Autodesk Inventor part; units mm, degrees
ref_plane "Work Plane1" through (0, -12.75, 0) normal (0, 1, 0) x (-1, 0, 0)
ref_plane "Work Plane2" through (0, -12.75, 0) normal (0, 1, 0) x (-1, 0, 0)
ref_plane "YZ Plane" through (0, 0, 0) normal (1, 0, 0) x (0, 1, 0)
sketch "Sketch1" plane through (0, 0, 0) normal (0, 0, 1) x (1, 0, 0)
  circle A0 centre (0, 0) radius 12.75
  circle A1 centre (0, 0) radius 12.25
  dimension "d0" = 25.5
  dimension "d1" = 24.5
extrude "Extrusion1" add sketch "Sketch1" along normal blind 49.5
sketch "Sketch2" plane through (0, 0, 49.5) normal (0, 0, 1) x (1, 0, 0)
  line L0 (-17.85, 0) -> (17.85, 0)
  line L1 (0, -17.85) -> (0, 17.85)
  line L2 (0, 0) -> (-12.3156, 3.2999)
  line L3 (0, 0) -> (-9.0156, -9.0156)
  line L4 (0, 0) -> (12.3156, 3.2999)
  line L5 (0, 0) -> (9.0156, -9.0156)
  arc A0 (11.8326, 3.1705) -> (-11.8326, 3.1705) centre (0, 0) ccw
  arc A1 (-8.6621, -8.6621) -> (8.6621, -8.6621) centre (0, 0) ccw
  circle A2 centre (0, 0) radius 12.75
  dimension "d4" = 15
  dimension "d5" = 45
extrude "Extrusion2" cut sketch "Sketch2" against normal blind 10 contours L5 A1 L1 | L1 A1 L3 | A1 L5 A2 L1 | L1 A2 L3 A1 | A0 L2 A2 L1 | L1 A2 L4 A0
sketch "Sketch3" plane through (0, 0, 0) normal (0, 0, -1) x (-1, 0, 0)
  circle A0 centre (0, 0) radius 12.75
extrude "Extrusion3" add sketch "Sketch3" along normal blind 1
ref_plane "Work Plane1" through (0, -12.75, 0) normal (0, 1, 0) x (-1, 0, 0)
ref_plane "Work Plane2" through (0, -12.75, 0) normal (0, 1, 0) x (-1, 0, 0)
sketch "Sketch7" plane through (0, 0, 49.5) normal (0, 0, 1) x (1, 0, 0)
  arc A0 (9.0156, -9.0156) -> (12.3156, 3.2999) centre (0, 0) ccw
  arc A1 (8.6621, -8.6621) -> (11.8326, 3.1705) centre (0, 0) ccw
  line L0 (8.6621, -8.6621) -> (9.0156, -9.0156)
  line L1 (-10.4211, -8.1317) -> (11.1081, -8.1317)
  line L2 (11.1081, -8.1317) -> (11.1081, -13.0652)
  line L3 (11.1081, -13.0652) -> (-10.4211, -13.0652)
  line L4 (-10.4211, -13.0652) -> (-10.4211, -8.1317)
extrude "Extrusion6" cut sketch "Sketch7" against normal through all
sketch "Sketch9" plane through (0, 0, 0) normal (0, 0, 1) x (1, 0, 0)
  arc A0 (9.1617, -8.1317) -> (-9.1617, -8.1317) centre (0, 0) ccw
  line L0 (-17.85, 0) -> (17.85, 0)
  point P0 (4, 0)
  dimension "d29" = 4
hole "Hole2" at (4, 0, 0) direction (0, 0, -1) diameter 1.778 depth 8 tip angle 118 countersink diameter 3.023 countersink angle 82
pattern_circular "Circular Pattern1" count 3 over 360 about axis through (0, 0, -10) along (0, 0, 1) of "Hole2"
sketch "Sketch10" plane through (0, 0, 0) normal (0, 0, 1) x (1, 0, 0)
  arc A0 (9.1617, -8.1317) -> (-9.1617, -8.1317) centre (0, 0) ccw
hole "Hole3" at (0, 0, 0) direction (0, 0, -1) diameter 1.778 end through all
properties part number "ss_inner_guide_top"
Input: part model. Units: mm. Frame: model coordinates. A direction names the side the tool comes from. Coordinates: 2 decimals unless noted, no trailing zeros. Loops run counter-clockwise (first coordinate to the right, second up) from the corner with the lowest first, then second, coordinate; pieces in that order, holes last. Notation, with made-up numbers: M 10.25,69 L 43.25,69 A15 ccw 43.25,78 Z; hole C 40,-1.75 d8. An arc over 180 degrees is marked long. Answer in a Markdown table with one row per item.
1. Section B-B, the plane x = 0. Output: boundary loops of the cut face in (y, z).
Response:
| item | result |
|---|---|
| outline | M -8.13,-1 L -0.89,-1 L -0.89,0 L -8.13,0 Z; M 0.89,-1 L 12.75,-1 L 12.75,39.5 L 12.25,39.5 L 12.25,0 L 0.89,0 Z |
2. Draft query along Y for faces 3 (the flat face through (12.1, -2.8, 49.5)), 4 (the cylindrical face through (0.404, 12.744, 24.604)), 5 (the cylindrical face through (0.87, 0.19, -0.51)), 6 (the flat face through (-9.5, -8.132, 24.4)). Return one class per face: pulls with the +Y half, pulls with the -Y half, needs draft (parallel to the pull), parting line crosses it, or undercut.
Response:
| item | result |
|---|---|
| face 3 | needs draft |
| face 4 | parting line crosses it |
| face 5 | undercut |
| face 6 | pulls with the -Y half |
3. Section C-C, the plane y = -6. Output: boundary loops of the cut face in (x, z).
Response:
| item | result |
|---|---|
| outline | M -11.25,-1 L 11.25,-1 L 11.25,49.5 L 10.68,49.5 L 10.68,0 L -10.68,0 L -10.68,49.5 L -11.25,49.5 Z |
4. Section D-D, the plane x = 4. Output: boundary loops of the cut face in (y, z), then the cut area to 3 significant figures.
Response:
| item | result |
|---|---|
| outline | M -8.13,-1 L -0.89,-1 L -0.89,-0.72 L -1.51,0 L -8.13,0 Z; M 0.89,-1 L 12.11,-1 L 12.11,39.5 L 11.58,39.5 L 11.58,0 L 1.51,0 L 0.89,-0.72 Z |
| area | 38.9 mm2 |
5. Material intervals for line 1 (Y direction, x = 0, z = -0.45); line 2 (X direction, y = 0.25, z = 7); line 3 (Z direction, x = 2, y = 11.25), sorted ascending.
Response:
| item | result |
|---|---|
| line 1 | y = -8.13 to -0.89, 0.89 to 12.75 |
| line 2 | x = -12.75 to -12.25, 12.25 to 12.75 |
| line 3 | z = -1 to 0 |
6. Reachability of faces 1 (the flat face through (0, 2, -1)), 2 (the cylindrical face through (-0.394, 12.244, 24.404)) from +Z, -Z, +X, -X, +Y, -Y: full face, straight path, thin tool, end or side. Return the list, or none.
Response:
| item | result |
|---|---|
| face 1 | -Z, +X, -X, +Y, -Y |
| face 2 | +Z |
7. First-contact query: pin 1 (1 mm diameter, centred on x = 2.5, z = 8, fed in from -Y); pin 2 (5 mm diameter, centred on x = -1.5, y = 0, fed in from +Z); pin 3 (10 mm diameter, centred on x = -1, z = 32, fed in from +Y); pin 4 (10 mm diameter, centred on x = -2.5, z = 34, fed in from -Y). Flat tips, straight axial feed; report the tip coordinate or a pass-through.
Response:
| item | result |
|---|---|
| pin 1 | stops at y = 11.88 |
| pin 2 | stops at z = 0 |
| pin 3 | stops at y = 12.75 |
| pin 4 | stops at y = 9.69 |
8. Section A-A, the plane y = 0. Output: boundary loops of the cut face in (x, z), then the cut area to 3 significant figures.
Response:
| item | result |
|---|---|
| outline | M -12.75,-1 L -0.89,-1 L -0.89,0 L -12.25,0 L -12.25,49.5 L -12.75,49.5 Z; M 0.89,-1 L 3.11,-1 L 3.11,-0.72 L 2.49,0 L 0.89,0 Z; M 4.89,-1 L 12.75,-1 L 12.75,49.5 L 12.25,49.5 L 12.25,0 L 5.51,0 L 4.89,-0.72 Z |
| area | 71.0 mm2 |
